```python
from build123d import *

# Parameters (mm, degrees)
CROQUIS1_R              = 3.975
SALIENTE_EXTRUIR1_DEPTH = 60
CORTAR_EXTRUIR1_START   = -4
CORTAR_EXTRUIR1_DEPTH   = 4


with BuildPart() as part:
    # Croquis1 → Saliente-Extruir1 (new body)
    with BuildSketch(Plane(origin=(0, 0, 0), x_dir=(1, 0, 0), z_dir=(0, 1, 0))):
        with Locations(Location((0, 0, 0), (0, 0, 270))):
            Circle(CROQUIS1_R)
    extrude(amount=SALIENTE_EXTRUIR1_DEPTH)

    # Croquis2 → Cortar-Revolución1 (revolve, cut)
    with BuildSketch(Plane.XY, mode=Mode.PRIVATE) as cortar_revoluci_n1_sk:
        with BuildLine():
            Line((3.975, 33.527120168), (3.975, 36.472879832))
            ThreePointArc((3.975, 36.472879832), (3, 35), (3.975, 33.527120168))
        make_face()
    revolve(cortar_revoluci_n1_sk.sketch.rotate(Axis((0, 0, 0), (0, 1, 0)), 90), axis=Axis((0, 0, 0), (0, 1, 0)), mode=Mode.SUBTRACT)

    # Croquis3 → Cortar-Extruir1 (cut)
    with BuildSketch(Plane(origin=(0, 60, 0), x_dir=(1, 0, 0), z_dir=(0, 1, 0)).offset(CORTAR_EXTRUIR1_START)):
        with BuildLine():
            Line((-2.607800798, 3), (2.607800798, 3))
            ThreePointArc((2.607800798, 3), (0, 3.975), (-2.607800798, 3))
        make_face()
        with BuildLine():
            Line((-2.607800798, -3), (2.607800798, -3))
            ThreePointArc((2.607800798, -3), (0, -3.975), (-2.607800798, -3))
        make_face()
    extrude(amount=CORTAR_EXTRUIR1_DEPTH, mode=Mode.SUBTRACT)


solid = part.part
```
Geometry check sheet. Reference: the model listing, model coordinates, mm. A direction names the side the tool comes from. Give positions to 0.01 mm unless a question says otherwise; leave off trailing zeros. Order: outer loops, then holes, each group sorted by start corner. A loop starts at its lowest first (then second) coordinate and runs counter-clockwise, first axis right, second up. Notation, with made-up numbers: (36, 6) - (58, 6) arc R20 cw to (58, 20) - close; hole circle Ø11 at (25, -23.75). An arc over 180 degrees is marked (long way). Write item = value, one per line. Start each with the question number.
1) Section check A-A (y = 48). Enter the section's corners in (x, z) (3 decimals), then the cut area to 3 significant figures.
2) Scan lines: L1, parallel to X at y = 10, z = -3; L2, parallel to Y at x = 0.5, z = 3.75. Record each from-to range of solid material in increasing order.
3) Gauge pin test, flat ends, axial feed: pin 1 Ø1.5 at (x, y) = (-2.5, 49.5) entering from +Z; pin 2 Ø2 at (x, y) = (-1, 58.5) entering from +Z; pin 3 Ø1 at (x, y) = (-3, 30.5) entering from -Z. Record the tip position at first contact, or that the pin passes through.
4) Access from +Z, -Z, +X, -X, +Y, -Y to the whole of each face (thin tool, end or side, straight path). Record for faces 1 (the flat face through (0, 56, 3.4)), 2 (the cylindrical face through (3.94, 48.07, -0.52)), 3 (the flat face through (0, 58, -3)).
Geometry check:
q1.outline = circle Ø7.95 at (0, 0)
q1.area = 49.6 mm2
q2.L1 = -2.61 to 2.61
q2.L2 = 0 to 33.62, 36.38 to 56
q3.pin_1 = 3.57
q3.pin_2 = 3
q3.pin_3 = -3.09
q4.face_1 = +Z, +X, -X, +Y
q4.face_2 = +Y, -Y
q4.face_3 = -Z, +X, -X, +Y
